Source: CAD feature listing. Evaluate the final solid. Frame: model axes, mm. Round coordinates to 2 decimals unless told otherwise and drop trailing zeros. Loops run counter-clockwise (first coordinate to the right, second up) from the corner with the lowest first, then second, coordinate; pieces in that order, holes last.
Item 1: Section query C-C on y = -3.75. Return loops of the section in (x, z).
Item 2: Section query B-B on z = 4.2. Return loops of the section in (x, y).
Item 3: Pull-direction query (X, two-part tool) for faces 1 (the flat face through (-1, 12.75, 2)), 2 (the cylindrical face through (62.352, 0.088, 2.535)), 3 (the flat face through (-69.35, 0, 2)); classes: released by +X, released by -X, zero draft, split by the parting line, or undercut.
Item 4: Section query A-A on x = -64.35. Return loops of the section in (y, z).
Item 5: Ray query, L1, parallel to X at y = 0.25, z = 4.1; L2, parallel to Y at x = 20, z = 3.15; L3, parallel to X at y = 3.25, z = 2.4. Return the intervals inside material, ascending.
```python
from build123d import *

# Parameters (mm, degrees)
F0_W     = 138.7
F0_H     = 25.5
F1_DEPTH = 5
F2_R     = 9.5
F3_DEPTH = 25
F5_R     = 2
F5_R_2   = 1.5
F6_DEPTH = 25


with BuildPart() as f1:
    # F0 (on Top) → F1 (new body)
    with BuildSketch(Plane.XY):
        Rectangle(F0_W, F0_H)
    extrude(amount=F1_DEPTH)

    # F2 (on face) → F3 (cut)
    with BuildSketch(Plane.XY.offset(5)):
        Circle(F2_R)
    extrude(amount=-F3_DEPTH, mode=Mode.SUBTRACT)

    # F5 (on face) → F6 (cut)
    with BuildSketch(Plane.XY.offset(5)):
        with Locations((-64.35, 0)):
            Circle(F5_R)
        with Locations((64.35, 0)):
            Circle(F5_R)
        with Locations((20, 0)):
            Circle(F5_R_2)
        with Locations((-20, 0)):
            Circle(F5_R_2)
    extrude(amount=-F6_DEPTH, mode=Mode.SUBTRACT)


solid = f1.part
```
Data:
1. outline: (-69.35, 0) - (-8.73, 0) - (-8.73, 5) - (-69.35, 5) - close; (8.73, 0) - (69.35, 0) - (69.35, 5) - (8.73, 5) - close
2. outline: (-69.35, -12.75) - (69.35, -12.75) - (69.35, 12.75) - (-69.35, 12.75) - close; hole circle Ø4 at (-64.35, 0); hole circle Ø3 at (-20, 0); hole circle Ø19 at (0, 0); hole circle Ø3 at (20, 0); hole circle Ø4 at (64.35, 0)
3. face 1: zero draft
3. face 2: undercut
3. face 3: released by -X
4. outline: (-12.75, 0) - (-2, 0) - (-2, 5) - (-12.75, 5) - close; (2, 0) - (12.75, 0) - (12.75, 5) - (2, 5) - close
5. L1: x = -69.35 to -66.33, -62.37 to -21.48, -18.52 to -9.5, 9.5 to 18.52, 21.48 to 62.37, 66.33 to 69.35
5. L2: y = -12.75 to -1.5, 1.5 to 12.75
5. L3: x = -69.35 to -8.93, 8.93 to 69.35
